Check sheet for the modelled part. Datum: model origin and axes. Units: mm. A direction names the side the tool comes from. Round coordinates to 2 decimals unless told otherwise and drop trailing zeros. Write each loop counter-clockwise with the first axis right and the second up, starting at its lowest first coordinate (ties: lowest second). Pieces come first, ordered by that corner, then holes.
Item 1: Section check C-C, the plane y = -5. State how many separate pieces and enclosed holes the cut face has, plus the area to 3 significant figures.
Item 2: Section check B-B, the plane x = 37.5. Record the cut outline in (y, z), plus the area to 3 significant figures.
Item 3: Set-up check for faces 3 (the cylindrical face through (88.93, -23.133, -10.849)), 4 (the flat face through (32, -10, 4.965)): record each of +Z, -Z, +X, -X, +Y, -Y from which the full face is reachable in a straight line by a thin tool's end or side.
Item 4: Material ranges on line 1 along X through (y, z) = (-4, -5.5); line 2 along Z through (x, y) = (-50.5, -15); line 3 along Y through (x, z) = (69, 8), recorded low to high.
Item 5: Release check for a two-part mould opening along Z. For faces 1 (the flat face through (-33, -10, 4.867)), 2 (the flat face through (-1, -18, -21)) record: pulls with the +Z half, pulls with the -Z half, needs draft (parallel to the pull), parting line crosses it, or undercut.
Item 6: Depth check by flat-ended pin: pin 1 (1.7 mm diameter, centred on x = 32, z = 8, fed in from +Y); pin 2 (1 mm diameter, centred on x = -9, y = -4.5, fed in from -Z); pin 3 (2 mm diameter, centred on x = 58, y = -9.5, fed in from +Z). Enter the tip coordinate at first touch or a pass-through.
Item 7: Section check A-A, the plane z = -19. Record the cut outline in (x, y), plus the area to 3 significant figures.
Item 8: Section check D-D, the plane y = -29.5. Record the cut outline in (x, z), plus the area to 3 significant figures.
from build123d import *

# Parameters (mm, degrees)
SKETCH_1_W          = 195
SKETCH_1_H          = 72
EXTRUDE_1_DEPTH     = 3
SKETCH_2_W          = 168
SKETCH_2_H          = 42
EXTRUDE_2_DEPTH     = 40
SKETCH_2_2_W        = 168
SKETCH_2_2_H        = 42
CUT_EXTRUDE_1_DEPTH = 1
SKETCH_3_R          = 4
EXTRUDE_3_DEPTH     = 10
SKETCH_4_R          = 4
EXTRUDE_4_DEPTH     = 10
SKETCH_7_W          = 3.370643822
SKETCH_7_H          = 9.043190742
CUT_EXTRUDE_2_DEPTH = 25
SKETCH_6_W          = 3.579680374
SKETCH_6_H          = 9.801505786
CUT_EXTRUDE_3_DEPTH = 25
SKETCH_8_W          = 3.328212
SKETCH_8_H          = 8.8197618
CUT_EXTRUDE_4_DEPTH = 25


with BuildPart() as part:
    # 草图1 → 凸台-拉伸1 (new body)
    with BuildSketch(Plane(origin=(0, 0, 0), x_dir=(1, 0, 0), z_dir=(0, 1, 0))):
        Rectangle(SKETCH_1_W, SKETCH_1_H)
    extrude(amount=EXTRUDE_1_DEPTH)

    # 草图2 → 凸台-拉伸2 (add)
    with BuildSketch(Plane(origin=(0, 3, 0), x_dir=(1, 0, 0), z_dir=(0, 1, 0))):
        Rectangle(SKETCH_2_W, SKETCH_2_H)
    extrude(amount=-EXTRUDE_2_DEPTH)

    # 草图2<2> → 切除-拉伸1 (cut)
    with BuildSketch(Plane(origin=(0, 3, 0), x_dir=(1, 0, 0), z_dir=(0, 1, 0))):
        Rectangle(SKETCH_2_2_W, SKETCH_2_2_H)
    extrude(amount=-CUT_EXTRUDE_1_DEPTH, mode=Mode.SUBTRACT)

    # 草图3 → 凸台-拉伸3 (add)
    with BuildSketch(Plane(origin=(84, 0, 0), x_dir=(0, 0, -1), z_dir=(1, 0, 0))):
        with Locations((-12.009379944, -19.151607151)):
            Circle(SKETCH_3_R)
    extrude(amount=EXTRUDE_3_DEPTH)

    # 草图4 → 凸台-拉伸4 (add)
    with BuildSketch(Plane(origin=(84, 0, 0), x_dir=(0, 0, -1), z_dir=(1, 0, 0))):
        with Locations((11.71568974, -19.228280966)):
            Circle(SKETCH_4_R)
    extrude(amount=EXTRUDE_4_DEPTH)

    # 草图7 → 切除-拉伸2 (cut)
    with BuildSketch(Plane(origin=(0, 2, 0), x_dir=(1, 0, 0), z_dir=(0, 1, 0))):
        with Locations((-32.896346176, -9.388907812)):
            Rectangle(SKETCH_7_W, SKETCH_7_H)
        with Locations((-74.896346176, -9.388907812)):
            Rectangle(SKETCH_7_W, SKETCH_7_H)
        with Locations((9.103653824, -9.388907812)):
            Rectangle(SKETCH_7_W, SKETCH_7_H)
        with Locations((51.103653824, -9.388907812)):
            Rectangle(SKETCH_7_W, SKETCH_7_H)
    extrude(amount=-CUT_EXTRUDE_2_DEPTH, mode=Mode.SUBTRACT)

    # 草图6 → 切除-拉伸3 (cut)
    with BuildSketch(Plane(origin=(0, 2, 0), x_dir=(1, 0, 0), z_dir=(0, 1, 0))):
        with Locations((-20.841650073, 8.216489042)):
            Rectangle(SKETCH_6_W, SKETCH_6_H)
        with Locations((-62.841650073, 8.216489042)):
            Rectangle(SKETCH_6_W, SKETCH_6_H)
        with Locations((21.158349927, 8.216489042)):
            Rectangle(SKETCH_6_W, SKETCH_6_H)
        with Locations((63.158349927, 8.216489042)):
            Rectangle(SKETCH_6_W, SKETCH_6_H)
    extrude(amount=-CUT_EXTRUDE_3_DEPTH, mode=Mode.SUBTRACT)

    # 草图8 → 切除-拉伸4 (cut)
    with BuildSketch(Plane(origin=(0, 2, 0), x_dir=(1, 0, 0), z_dir=(0, 1, 0))):
        with Locations((-9.739053762, -9.375255868)):
            Rectangle(SKETCH_8_W, SKETCH_8_H)
        with Locations((-51.739053762, -9.375255868)):
            Rectangle(SKETCH_8_W, SKETCH_8_H)
        with Locations((32.260946238, -9.375255868)):
            Rectangle(SKETCH_8_W, SKETCH_8_H)
        with Locations((74.260946238, -9.375255868)):
            Rectangle(SKETCH_8_W, SKETCH_8_H)
    extrude(amount=-CUT_EXTRUDE_4_DEPTH, mode=Mode.SUBTRACT)


solid = part.part
Values found:
1. separate pieces: 1
1. enclosed holes: 12
1. area: 6,680 mm2
2. outline: (-37, -21) - (0, -21) - (0, -36) - (3, -36) - (3, -21) - (2, -21) - (2, 21) - (3, 21) - (3, 36) - (0, 36) - (0, 21) - (-37, 21) - close
2. area: 1,730 mm2
3. face 3: +X
3. face 4: +Y
4. line 1: x = -84 to -64.63, -61.05 to -22.63, -19.05 to 19.37, 22.95 to 61.37, 64.95 to 84
4. line 2: z = -21 to 4.97, 13.79 to 21
4. line 3: y = -37 to 2
5. face 1: undercut
5. face 2: pulls with the -Z half
6. pin 1: stops at y = -23
6. pin 2: stops at z = -21
6. pin 3: stops at z = 21
7. outline: (-97.5, 0) - (-84, 0) - (-84, -37) - (84, -37) - (84, 0) - (97.5, 0) - (97.5, 3) - (84, 3) - (84, 2) - (-84, 2) - (-84, 3) - (-97.5, 3) - close
7. area: 6,630 mm2
8. outline: (-84, -21) - (84, -21) - (84, 21) - (-84, 21) - close
8. area: 7,060 mm2
